from build123d import *

# Parameters (mm, degrees)
SKETCH2_R          = 1.7859375
SKETCH2_W          = 25.4
SKETCH2_H          = 31.75
CUT_EXTRUDE1_DEPTH = 7.3025


with BuildPart() as part:
    # Sketch1 → Revolve1 (revolve)
    with BuildSketch(Plane(origin=(0, 0, 0), x_dir=(1, 0, 0), z_dir=(0, 1, 0)), mode=Mode.PRIVATE) as revolve1_sk:
        Polygon((0, 0), (-11.7, 0), (-11.7, 4.7625), (-12.7, 4.7625), (-12.7, 7.3025), (-9.16, 7.3025), (-9.16, 2.54), (0, 2.54), align=None)
    revolve(revolve1_sk.sketch.rotate(Axis((-16.7, 0, -8.744517985), (0, 0, 1)), 180), axis=Axis((-16.7, 0, -8.744517985), (0, 0, 1)))

    # Sketch2 → Cut-Extrude1 (cut)
    with BuildSketch(Plane(origin=(0, 0, -7.3025), x_dir=(-1, 0, 0), z_dir=(0, 0, -1))):
        with Locations((16.7, -12.7)):
            Circle(SKETCH2_R)
        with Locations((16.7, 12.7)):
            Circle(SKETCH2_R)
        with Locations((38.925, 0)):
            Rectangle(SKETCH2_W, SKETCH2_H)
        with Locations((-5.525, 0)):
            Rectangle(SKETCH2_W, SKETCH2_H)
    extrude(amount=-CUT_EXTRUDE1_DEPTH, mode=Mode.SUBTRACT)


solid = part.part
Here's how the part is built. I have some questions about the finished solid (model axes, mm). A direction names the side the tool comes from. Round coordinates to 2 decimals unless told otherwise and drop trailing zeros. Loops run counter-clockwise (first coordinate to the right, second up) from the corner with the lowest first, then second, coordinate; pieces in that order, holes last.
1. If we section it at B-B on x = -16.7: Write out the boundary of the cut face in (y, z), plus the area to 3 significant figures.
Answer list:
outline: (-16.7, -2.54) - (-14.49, -2.54) - (-14.49, 0) - (-16.7, 0) - close; (-10.91, -2.54) - (-7.54, -2.54) - (-7.54, -7.3) - (-4, -7.3) - (-4, -4.76) - (-5, -4.76) - (-5, 0) - (-10.91, 0) - close; (4, -7.3) - (7.54, -7.3) - (7.54, -2.54) - (10.91, -2.54) - (10.91, 0) - (5, 0) - (5, -4.76) - (4, -4.76) - close; (14.49, -2.54) - (16.7, -2.54) - (16.7, 0) - (14.49, 0) - close
area: 70.6 mm2
2. If we section it at C-C on z = -1.5: Write out the boundary of the cut face in (x, y) (3 decimals), plus the area to 3 significant figures.
Answer list:
outline: (-26.225, -13.717) arc R16.7 ccw to (-7.175, -13.717) - (-7.175, 13.717) arc R16.7 ccw to (-26.225, 13.717) - close; hole circle Ø10 at (-16.7, 0); hole circle Ø3.572 at (-16.7, -12.7); hole circle Ø3.572 at (-16.7, 12.7)
area: 501 mm2
3. We'd pull the mould along Y, two halves only. Please class faces 1 (the face through (-18.35, 12.02, -1.29)), 2 (the face through (-17, -8, -2.54)), 3 (the face through (-16.6, 16.7, -1.3)): +Y half, -Y half, draft (parallel to the pull), parting line (faces both ways), or undercut.
Answer list:
face 1: undercut
face 2: draft
face 3: +Y half
4. If I drill on line 1 along Y through (x, z) = (-16.7, -6.55); line 2 along Y through (x, z) = (-16.7, -1.95); line 3 along Y through (x, z) = (-18, -2), over which ranges is the centre line in solid material (lowest first)?
Answer list:
line 1: y = -7.54 to -4, 4 to 7.54
line 2: y = -16.7 to -14.49, -10.91 to -5, 5 to 10.91, 14.49 to 16.7
line 3: y = -16.65 to -13.92, -11.48 to -4.83, 4.83 to 11.48, 13.92 to 16.65
5. If we section it at D-D on y = 0: Write out the boundary of the cut face in (x, z) (1 decimal).
Answer list:
outline: (-26.2, -2.5) - (-24.2, -2.5) - (-24.2, -7.3) - (-20.7, -7.3) - (-20.7, -4.8) - (-21.7, -4.8) - (-21.7, 0) - (-26.2, 0) - close; (-12.7, -7.3) - (-9.2, -7.3) - (-9.2, -2.5) - (-7.2, -2.5) - (-7.2, 0) - (-11.7, 0) - (-11.7, -4.8) - (-12.7, -4.8) - close
6. For P1, Ø4, axis at x = -16.7, y = 12.7, coming from the -Z side; P2, Ø3, axis at x = -14.5, z = -1, coming from the -Y side; P3, Ø4, axis at y = 5, z = -5.5, coming from the -X side; P4, Ø3, axis at x = -16.7, y = -12.7, coming from the -Z side, each with a flat end and sliding along its axis, tell me the tip position at first contact or that it passes through.
Answer list:
P1: stops at z = -2.54
P2: stops at y = -16.69
P3: stops at x = -23.62
P4: passes through
7. If we section it at A-A on y = -12.7: Write out the boundary of the cut face in (x, z) (3 decimals), plus the area to 3 significant figures.
Answer list:
outline: (-26.225, -2.54) - (-18.486, -2.54) - (-18.486, 0) - (-26.225, 0) - close; (-14.914, -2.54) - (-7.175, -2.54) - (-7.175, 0) - (-14.914, 0) - close
area: 39.3 mm2
8. Which directions (+Z, -Z, +X, -X, +Y, -Y) give clear straight access to the entire face, cutting with the end or side of a thin tool? Please do faces 4 (the face through (-23.665, 2.888, -4.888)), 5 (the face through (-11.705, -0.22, -2.415)), 6 (the face through (-26.225, 0, -1)).
Answer list:
face 4: -Z
face 5: +Z
face 6: +Z, -Z, -X, +Y, -Y
